Can you work these out from the model? Positions are in its coordinate system, mm. A direction names the side the tool comes from. Coordinates: 2 decimals unless noted, no trailing zeros. Order: outer loops, then holes, each group sorted by start corner. A loop starts at its lowest first (then second) coordinate and runs counter-clockwise, first axis right, second up. Notation, with made-up numbers: (-1.5, -35.75) -> (33.5, -35.75) arc R21 cw to (33.5, -15.75) -> close; hole circle Ø5 at (-5, -1). An arc over 180 degrees is marked (long way). Answer as a JSON object with one key per item and string values. Group by question number.
(1) I need wall thicknesses on line 1 (X direction, y = -8, z = 2.6); line 2 (Y direction, x = 25, z = 4.7); line 3 (Y direction, x = -1, z = 1.8). Which ranges of each line are inside material? Lowest first, please.
(2) I want a section at A-A, the plane z = 3.05. List the corners of the cut face in (x, y) for me, plus the area to 3 significant figures.
(3) For pin 1 (2.5 mm diameter, centred on y = 28, z = 3.5, fed in from -X); pin 2 (2.5 mm diameter, centred on y = -24.5, z = 2.5, fed in from +X); pin 3 (2.5 mm diameter, centred on x = -25, z = 1.5, fed in from +Y), each with a flat end and sliding along its axis, tell me the tip position at first contact or that it passes through.
(4) Which directions (+Z, -Z, +X, -X, +Y, -Y) give clear straight access to the entire face, cutting with the end or side of a thin tool? Please do faces 1 (the flat face through (27, 7.5, 2)), 2 (the flat face through (22.5, -29, 2)), 3 (the flat face through (-26, 7.5, 2)), 4 (the flat face through (-27, -7.5, 2)).
(5) I want a section at B-B, the plane y = -5.5. List the corners of the cut face in (x, z) for me, plus the area to 3 significant figures.
(6) I want a section at D-D, the plane y = 17. List the corners of the cut face in (x, z) for me.
(7) I want a section at C-C, the plane x = 2.5. List the corners of the cut face in (y, z) for me.
from build123d import *

# Parameters (mm, degrees)
F1_DEPTH = 5


with BuildPart() as f1:
    # F0 (on Top) → F1 (new body)
    with BuildSketch(Plane.XY):
        with BuildLine():
            Line((-22.5, 7.5), (-30.5, 7.5))
            Line((-30.5, 7.5), (-30.5, -7.5))
            Line((-30.5, -7.5), (-22.5, -7.5))
            Line((-22.5, -7.5), (-22.5, -50))
            Line((-22.5, -50), (0, -50))
            Line((0, -50), (0, -7))
            ThreePointArc((0, -7), (-7, 0), (0, 7))
            Line((0, 7), (0, 50))
            Line((0, 50), (-22.5, 50))
            Line((-22.5, 50), (-22.5, 7.5))
        make_face()
        with BuildLine():
            Line((22.5, 50), (0, 50))
            Line((0, 50), (0, 7))
            ThreePointArc((0, 7), (4.949747, 4.949747), (7, 0))
            ThreePointArc((7, 0), (4.949747, -4.949747), (0, -7))
            Line((0, -7), (0, -50))
            Line((0, -50), (22.5, -50))
            Line((22.5, -50), (22.5, -7.5))
            Line((22.5, -7.5), (30.5, -7.5))
            Line((30.5, -7.5), (30.5, 7.5))
            Line((30.5, 7.5), (22.5, 7.5))
            Line((22.5, 7.5), (22.5, 50))
        make_face()
    extrude(amount=F1_DEPTH)


solid = f1.part
Computed values:
{
 "1": {"line 1": "x = -22.5 to 22.5", "line 2": "y = -7.5 to 7.5", "line 3": "y = -50 to -6.93, 6.93 to 50"},
 "2": {"outline": "(-30.5, -7.5) -> (-22.5, -7.5) -> (-22.5, -50) -> (22.5, -50) -> (22.5, -7.5) -> (30.5, -7.5) -> (30.5, 7.5) -> (22.5, 7.5) -> (22.5, 50) -> (-22.5, 50) -> (-22.5, 7.5) -> (-30.5, 7.5) -> close; hole (0, -7) arc R7 ccw to (7, 0) arc R7 ccw to (0, 7) arc R7 ccw to start", "area": "4,590 mm2"},
 "3": {"pin 1": "stops at x = -22.5", "pin 2": "stops at x = 22.5", "pin 3": "stops at y = 7.5"},
 "4": {"face 1": "+Z, -Z, +X, +Y", "face 2": "+Z, -Z, +X, -Y", "face 3": "+Z, -Z, -X, +Y", "face 4": "+Z, -Z, -X, -Y"},
 "5": {"outline": "(-30.5, 0) -> (-4.33, 0) -> (-4.33, 5) -> (-30.5, 5) -> close; (4.33, 0) -> (30.5, 0) -> (30.5, 5) -> (4.33, 5) -> close", "area": "262 mm2"},
 "6": {"outline": "(-22.5, 0) -> (22.5, 0) -> (22.5, 5) -> (-22.5, 5) -> close"},
 "7": {"outline": "(-50, 0) -> (-6.54, 0) -> (-6.54, 5) -> (-50, 5) -> close; (6.54, 0) -> (50, 0) -> (50, 5) -> (6.54, 5) -> close"}
}
